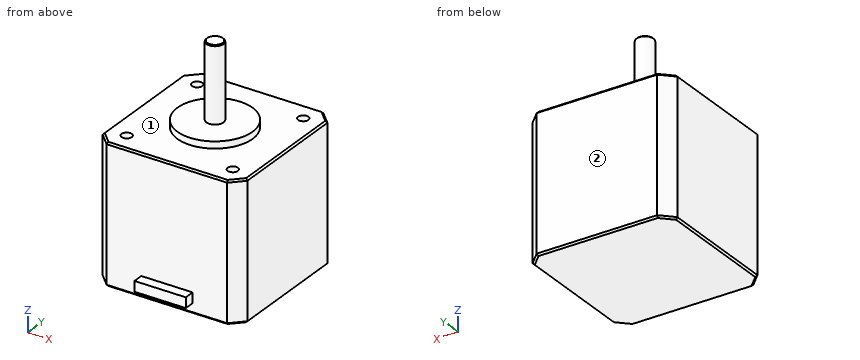
```python
from build123d import *

# Parameters (mm, degrees)
PAD_DEPTH       = 40
SKETCH002_R     = 2.5
PAD001_DEPTH    = 24
SKETCH001_R     = 11
PAD002_DEPTH    = 2
SKETCH003_R     = 1.5
POCKET_DEPTH    = 5
CHAMFER_SIZE    = 0.5
CHAMFER001_SIZE = 0.25
SKETCH004_W     = 15
SKETCH004_H     = 3
PAD003_DEPTH    = 3


with BuildPart() as part:
    # Sketch → Pad (new body)
    with BuildSketch(Plane.XY):
        Polygon((-17.614466, 21.15), (17.614466, 21.15), (21.15, 17.614466), (21.15, -17.614466), (17.614466, -21.15), (-17.614466, -21.15), (-21.15, -17.614466), (-21.15, 17.614466), align=None)
    extrude(amount=PAD_DEPTH)

    # Sketch002 (on Face10 of Pad) → Pad001 (join)
    with BuildSketch(Plane.XY.offset(40)):
        Circle(SKETCH002_R)
    extrude(amount=PAD001_DEPTH)

    # Sketch001 (on Face10 of Pad) → Pad002 (join)
    with BuildSketch(Plane.XY.offset(40)):
        Circle(SKETCH001_R)
    extrude(amount=PAD002_DEPTH)

    # Sketch003 (on Face5 of Pad002) → Pocket (cut)
    with BuildSketch(Plane.XY.offset(40)):
        with Locations((-15.5, 15.5)):
            Circle(SKETCH003_R)
        with Locations((15.5, 15.5)):
            Circle(SKETCH003_R)
        with Locations((-15.5, -15.5)):
            Circle(SKETCH003_R)
        with Locations((15.5, -15.5)):
            Circle(SKETCH003_R)
    extrude(amount=-POCKET_DEPTH, mode=Mode.SUBTRACT)

    # Chamfer
    chamfer_edges = [part.edges().sort_by_distance(p)[0] for p in [
        (-19.382233, 19.382233, 0),
        (0, 21.15, 0),
        (19.382233, 19.382233, 0),
        (21.15, 0, 0),
        (19.382233, -19.382233, 0),
        (0, -21.15, 0),
        (-19.382233, -19.382233, 0),
        (-21.15, 0, 0),
        (0, -21.15, 40),
        (21.15, 0, 40),
        (19.382233, -19.382233, 40),
        (19.382233, 19.382233, 40),
        (0, 21.15, 40),
        (-19.382233, -19.382233, 40),
        (-21.15, 0, 40),
        (-19.382233, 19.382233, 40),
    ]]
    chamfer(chamfer_edges, length=CHAMFER_SIZE)

    # Chamfer001
    chamfer001_edges = [part.edges().sort_by_distance(p)[0] for p in [
        (-2.5, 0, 64),
    ]]
    chamfer(chamfer001_edges, length=CHAMFER001_SIZE)

    # Sketch004 (on Face19 of Chamfer001) → Pad003 (join)
    with BuildSketch(Plane.XZ.offset(21.15)):
        with Locations((0, 4.5)):
            Rectangle(SKETCH004_W, SKETCH004_H)
    extrude(amount=PAD003_DEPTH)


solid = part.part
```
Input: part model. Units: mm. Frame: model coordinates. Face numbers are marked on the shaded views. A direction names the side the tool comes from. Coordinates: 2 decimals unless noted, no trailing zeros. Write each loop counter-clockwise with the first axis right and the second up, starting at its lowest first coordinate (ties: lowest second). Pieces come first, ordered by that corner, then holes. Notation, with made-up numbers: (-1.75, -3) - (29.25, -3) arc R19 cw to (29.25, 33) - close; hole circle Ø1 at (14, 2.5). An arc over 180 degrees is marked (long way). Put each result on its own line as item: value. Start each with the question number.
1) Ray query, L1, parallel to Y at x = -15.5, z = 38.15; L2, parallel to Y at x = 15, z = 38. Return the intervals inside material, ascending.
2) Cut plane C-C (x = 0). Return the cut outline in (y, z), plus the area to 3 significant figures.
3) Contact query for flat-ended pins moving along their axis: pin 1 (3.5 mm diameter, centred on y = -22.5, z = 4.5, fed in from -X); pin 2 (24 mm diameter, centred on x = 3.5, y = 2, fed in from +Z); pin 3 (3.5 mm diameter, centred on x = -3, y = -23, fed in from +Z); pin 4 (3 mm diameter, centred on x = 0.5, z = 8, fed in from -Y). Output: stop coordinate, or through.
4) Reachability of the marked faces 1 and 2 from +Z, -Z, +X, -X, +Y, -Y: full face, straight path, thin tool, end or side. Return the list, or none.
5) Cut plane A-A (x = -15.5). Return the cut outline in (y, z).
6) Cut plane B-B (y = 0). Return the cut outline in (x, z), plus the area to 3 significant figures.
Resolved:
1. L1: y = -21.15 to -17, -14 to 14, 17 to 21.15
1. L2: y = -21.15 to -16.91, -14.09 to 14.09, 16.91 to 21.15
2. outline: (-24.15, 3) - (-21.15, 3) - (-21.15, 0.5) - (-20.65, 0) - (20.65, 0) - (21.15, 0.5) - (21.15, 39.5) - (20.65, 40) - (11, 40) - (11, 42) - (2.5, 42) - (2.5, 63.75) - (2.25, 64) - (-2.25, 64) - (-2.5, 63.75) - (-2.5, 42) - (-11, 42) - (-11, 40) - (-20.65, 40) - (-21.15, 39.5) - (-21.15, 6) - (-24.15, 6) - close
2. area: 1,850 mm2
3. pin 1: stops at x = -18.01
3. pin 2: stops at z = 64
3. pin 3: stops at z = 6
3. pin 4: stops at y = -21.15
4. face 1: +Z
4. face 2: +Z, -Z, +X, -X, +Y
5. outline: (-21.15, 0.5) - (-20.65, 0) - (20.65, 0) - (21.15, 0.5) - (21.15, 39.5) - (20.65, 40) - (17, 40) - (17, 35) - (14, 35) - (14, 40) - (-14, 40) - (-14, 35) - (-17, 35) - (-17, 40) - (-20.65, 40) - (-21.15, 39.5) - close
6. outline: (-21.15, 0.5) - (-20.65, 0) - (20.65, 0) - (21.15, 0.5) - (21.15, 39.5) - (20.65, 40) - (11, 40) - (11, 42) - (2.5, 42) - (2.5, 63.75) - (2.25, 64) - (-2.25, 64) - (-2.5, 63.75) - (-2.5, 42) - (-11, 42) - (-11, 40) - (-20.65, 40) - (-21.15, 39.5) - close
6. area: 1,850 mm2
